Part model, mm, in its own coordinate system. A direction names the side the tool comes from. Give positions to 0.01 mm unless a question says otherwise; leave off trailing zeros. Order: outer loops, then holes, each group sorted by start corner. A loop starts at its lowest first (then second) coordinate and runs counter-clockwise, first axis right, second up. Notation, with made-up numbers: M 58.5,29 L 117.5,29 A29 ccw 117.5,59 Z; hole C -2,41 d3. An arc over 180 degrees is marked long. One line per question, with ' | ' between items.
Autodesk Inventor part; units mm, degrees
ref_plane "YZ Plane" through (0, 0, 0) normal (1, 0, 0) x (0, 1, 0)
ref_plane "XZ Plane" through (0, 0, 0) normal (0, 1, 0) x (-1, 0, 0)
ref_plane "XY Plane" through (0, 0, 0) normal (0, 0, 1) x (1, 0, 0)
sketch "Skizze1" plane through (0, 0, 0) normal (0, 1, 0) x (-1, 0, 0)
  circle A0 centre (0, 0) radius 6.5
  dimension "d0" = 13
extrude "Extrusion1" add sketch "Skizze1" along normal blind 2
sketch "Skizze2" plane through (0, 2, 0) normal (0, 1, 0) x (1, 0, 0)
  circle A0 centre (0, 0) radius 5
  circle A1 centre (0, 0) radius 6.5
  dimension "d3" = 10
  dimension "d4" = 13
extrude "Extrusion2" add sketch "Skizze2" along normal blind 2.5
sketch "Skizze3" plane through (0, 0, 0) normal (0, -1, 0) x (1, 0, 0)
  circle A0 centre (0, 0) radius 1.6
  dimension "d7" = 3.2
extrude "Extrusion3" cut sketch "Skizze3" against normal up to surface (2 mm away)
properties part number "Gegenstück_Welle_Diff"
1. Slice it at A-A on y = 3.2. Give the cut face in (x, z), then the cut area to 3 significant figures.
Worked out:
outline: C 0,0 d13; hole C 0,0 d10 | area: 54.2 mm2
2. Slice it at C-C on z = -4.25. Give the cut face in (x, y), then the cut area to 3 significant figures.
Worked out:
outline: M -4.92,0 L 4.92,0 L 4.92,4.5 L 2.63,4.5 L 2.63,2 L -2.63,2 L -2.63,4.5 L -4.92,4.5 Z | area: 31.1 mm2
3. Tool access for faces 4 (the cylindrical face through (-1.27, 0.99, -0.97)), 5 (the flat face through (-2, 2, 0)): list every direction of +Z, -Z, +X, -X, +Y, -Y with a clear straight run to the whole face (end or side of a thin tool).
Worked out:
face 4: +Y, -Y | face 5: +Y
4. Slice it at D-D on y = 0.6. Give the cut face in (x, z).
Worked out:
outline: C 0,0 d13; hole C 0,0 d3.2
5. Mould opens along Z. For faces 1 (the cylindrical face through (-1.08, 3.23, -4.88)), 2 (the flat face through (-1.4, 0, -1.4)), 3 (the cylindrical face through (0.429, 2.218, 6.486)) say: released by +Z, released by -Z, zero draft, split by the parting line, or undercut.
Worked out:
face 1: undercut | face 2: zero draft | face 3: split by the parting line
6. Drop flat-ended pins along their axis: pin 1 (2 mm diameter, centred on x = -4.5, y = 2, fed in from -Z); pin 2 (3.5 mm diameter, centred on x = 0, z = 0, fed in from +Y); pin 3 (2 mm diameter, centred on y = 0.5, z = 1, fed in from +X). Give the stop position or say it passes through.
Worked out:
pin 1: stops at z = -5.48 | pin 2: stops at y = 2 | pin 3: stops at x = 6.5
7. Probe L1, parallel to Z at x = 0, y = 3.9; L2, parallel to Z at x = 0, y = 1.4. List the from-to ranges inside material, lowest first. Write a range as from..to.
Worked out:
L1: z = -6.5..-5, 5..6.5 | L2: z = -6.5..-1.6, 1.6..6.5
